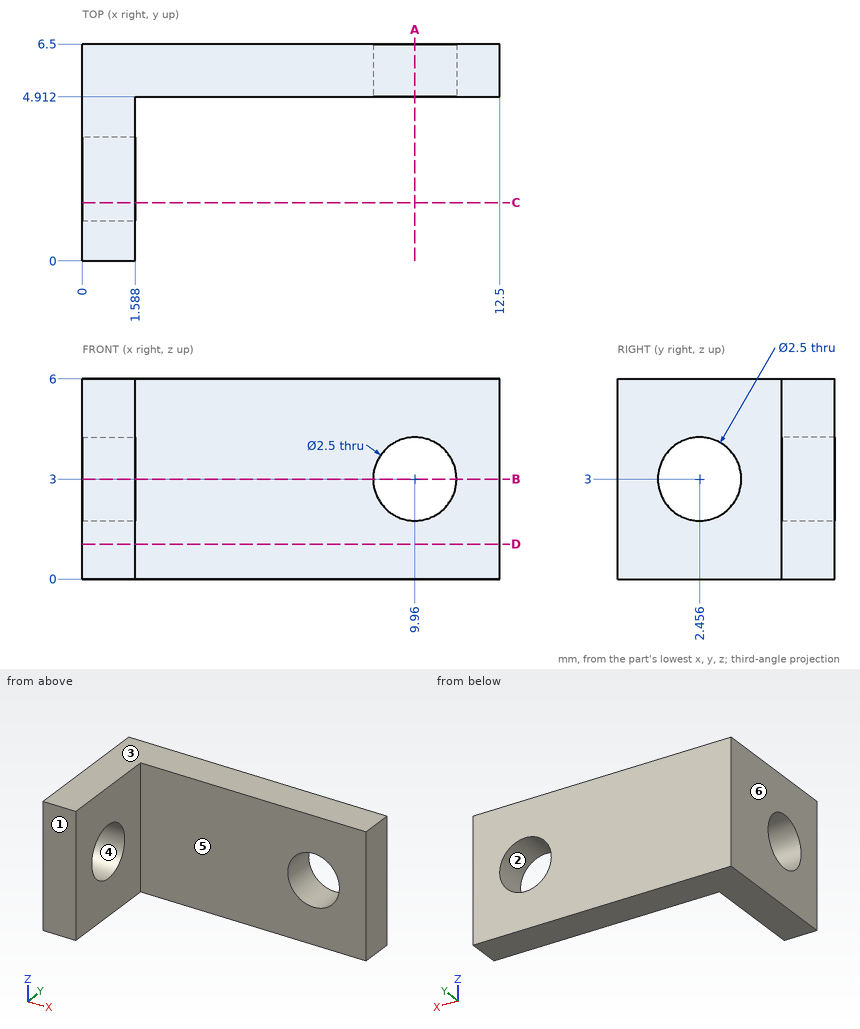
Verification items for this drawing (mm, ordinates from the low corner). A direction names the side the tool comes from. Coordinates: 2 decimals unless noted, no trailing zeros. Order: outer loops, then holes, each group sorted by start corner. A loop starts at its lowest first (then second) coordinate and runs counter-clockwise, first axis right, second up.
Q1. Draft check along Z on the marked faces 1, 2, 3 and 4. Enter one of: released by +Z, released by -Z, zero draft, split by the parting line, or undercut.
Reply:
face 1: zero draft
face 2: undercut
face 3: released by +Z
face 4: undercut
Q2. Tool access check on the marked faces 5 and 6. Record the directions out of +Z, -Z, +X, -X, +Y, -Y that give a thin tool (end or side, any length) a straight path to the whole face; none if there is none.
Reply:
face 5: +Z, -Z, +X, -Y
face 6: +Z, -Z, -X, +Y, -Y
Q3. Sectioned sample at C-C on y = 1.75. Record the cut outline in (x, z).
Reply:
outline: (0, 0) - (1.59, 0) - (1.59, 1.97) - (0, 1.97) - close; (0, 4.03) - (1.59, 4.03) - (1.59, 6) - (0, 6) - close
Q4. Sectioned sample at A-A on x = 9.96. Record the cut outline in (y, z).
Reply:
outline: (4.91, 0) - (6.5, 0) - (6.5, 1.75) - (4.91, 1.75) - close; (4.91, 4.25) - (6.5, 4.25) - (6.5, 6) - (4.91, 6) - close
Q5. Sectioned sample at D-D on z = 1.05. Record the cut outline in (x, y).
Reply:
outline: (0, 0) - (1.59, 0) - (1.59, 4.91) - (12.5, 4.91) - (12.5, 6.5) - (0, 6.5) - close
Q6. Thickness scan on probe 1 along X at (y, z) = (5.5, 3); probe 2 along Y at (x, z) = (8.25, 0.5); probe 3 along Z at (x, y) = (10.5, 5.25). Record the ranges inside material, lowest first.
Reply:
probe 1: x = 0 to 8.71, 11.21 to 12.5
probe 2: y = 4.91 to 6.5
probe 3: z = 0 to 1.87, 4.13 to 6
Q7. Sectioned sample at B-B on z = 3. Record the cut outline in (x, y), and give its area (3 significant figures).
Reply:
outline: (0, 0) - (1.59, 0) - (1.59, 1.21) - (0, 1.21) - close; (0, 3.71) - (1.59, 3.71) - (1.59, 4.91) - (8.71, 4.91) - (8.71, 6.5) - (0, 6.5) - close; (11.21, 4.91) - (12.5, 4.91) - (12.5, 6.5) - (11.21, 6.5) - close
area: 19.7 mm2
Q8. Depth check by flat-ended pin: pin 1 Ø1.5 at (y, z) = (1, 2) entering from +X; pin 2 Ø3 at (x, z) = (9.96, 3) entering from -Y. Enter the tip coordinate at first touch or a pass-through.
Reply:
pin 1: stops at x = 1.59
pin 2: stops at y = 4.91
